from build123d import *

# Parameters (mm, degrees)
SKETCH_1_W          = 10
SKETCH_1_H          = 10
SKETCH_1_W_2        = 8
SKETCH_1_H_2        = 8
EXTRUDE_1_DEPTH     = 312
SKETCH_2_R          = 2
CUT_EXTRUDE_1_DEPTH = 313.200256246
SKETCH_3_R          = 2
CUT_EXTRUDE_2_DEPTH = 313.200256246


with BuildPart() as part:
    # ｽｹｯﾁ1 → 押し出し-薄板1 (new body)
    with BuildSketch(Plane(origin=(0, 0, 0), x_dir=(0, 0, -1), z_dir=(1, 0, 0))):
        Rectangle(SKETCH_1_W, SKETCH_1_H)
        Rectangle(SKETCH_1_W_2, SKETCH_1_H_2, mode=Mode.SUBTRACT)
    extrude(amount=EXTRUDE_1_DEPTH)

    # ｽｹｯﾁ2 → ｶｯﾄ - 押し出し1 (cut, through all)
    with BuildSketch(Plane(origin=(0, 5, 0), x_dir=(1, 0, 0), z_dir=(0, 1, 0))):
        with Locations(Location((5, 0, 0), (0, 0, 270))):
            Circle(SKETCH_2_R)
        with Locations(Location((307, 0, 0), (0, 0, 270))):
            Circle(SKETCH_2_R)
    extrude(amount=-CUT_EXTRUDE_1_DEPTH, mode=Mode.SUBTRACT)

    # ｽｹｯﾁ3 → ｶｯﾄ - 押し出し2 (cut, through all)
    with BuildSketch(Plane.XY.offset(5)):
        with Locations((136, 0)):
            Circle(SKETCH_3_R)
        with Locations((156, 0)):
            Circle(SKETCH_3_R)
        with Locations((176, 0)):
            Circle(SKETCH_3_R)
    extrude(amount=-CUT_EXTRUDE_2_DEPTH, mode=Mode.SUBTRACT)


solid = part.part
Work out the finished part from the listing and answer in its coordinate system (mm). A direction names the side the tool comes from. Coordinates: 2 decimals unless noted, no trailing zeros. Loops run counter-clockwise (first coordinate to the right, second up) from the corner with the lowest first, then second, coordinate; pieces in that order, holes last. Notation, with made-up numbers: M 30.25,10 L 78.25,10 A31 cw 78.25,34 Z; hole C 28,-18 d10. An arc over 180 degrees is marked long. Answer in a Markdown table with one row per item. Add a question column.
1. Consider L1, parallel to X at y = 4.65, z = 0; L2, parallel to Z at x = 142.5, y = -3.75. Determine where each line is inside the solid, lowest interval first.
2. Find section A-A, the plane z = 0. Write down the section's boundary in (x, y), then the cut area to 3 significant figures.
3. Find section B-B, the plane x = 86.5. Write down the section's boundary in (y, z).
4. A tool of negligible diameter and unlimited length cuts with its end or side. For faces 1 (the flat face through (312, 0.1, 4.5)), 2 (the flat face through (153.8, -0.1, -4)), from which of +Z, -Z, +X, -X, +Y, -Y can it reach the whole face along a straight path? Write none if from no direction.
5. The mould has two halves that part along Y. Classify faces 3 (the flat face through (153.8, -0.1, -5)), 4 (the flat face through (154, 5, 0)), 5 (the flat face through (153.8, -0.1, 4)), 6 (the flat face through (154, 4, 0)): pulls with the +Y half, pulls with the -Y half, needs draft (parallel to the pull), parting line crosses it, or undercut.
6. A flat-ended cylindrical pin translates along its axis: P1, Ø2, axis at y = 2, z = 1.5, coming from the +X side. Find the tip coordinate at first contact, or state that the pin passes through.
Reported:
| question | item | result |
|---|---|---|
| 1 | L1 | x = 0 to 3, 7 to 305, 309 to 312 |
| 1 | L2 | z = -5 to -4, 4 to 5 |
| 2 | outline | M 0,-5 L 3,-5 L 3,-4 L 0,-4 Z; M 0,4 L 3,4 L 3,5 L 0,5 Z; M 7,-5 L 305,-5 L 305,-4 L 7,-4 Z; M 7,4 L 305,4 L 305,5 L 7,5 Z; M 309,-5 L 312,-5 L 312,-4 L 309,-4 Z; M 309,4 L 312,4 L 312,5 L 309,5 Z |
| 2 | area | 608 mm^2 |
| 3 | outline | M -5,-5 L 5,-5 L 5,5 L -5,5 Z; hole M -4,-4 L 4,-4 L 4,4 L -4,4 Z |
| 4 | face 1 | +Z, -Z, +X, +Y, -Y |
| 4 | face 2 | +X, -X |
| 5 | face 3 | needs draft |
| 5 | face 4 | pulls with the +Y half |
| 5 | face 5 | undercut |
| 5 | face 6 | undercut |
| 6 | P1 | passes through |
